from build123d import *

# Parameters (mm, degrees)
F0_W     = 38.1
F0_H     = 38.1
F1_DEPTH = 38.1
F2_W     = 38.1
F2_H     = 36.83
F3_DEPTH = 36.83
F6_DEPTH = 3.81
F7_DEPTH = 4.826


with BuildPart() as f1:
    # F0 (on Top) → F1 (new body)
    with BuildSketch(Plane.XY):
        Rectangle(F0_W, F0_H)
    extrude(amount=F1_DEPTH)

    # F2 (on face) → F3 (cut)
    with BuildSketch(Plane.XY.offset(38.1)):
        with Locations((0, -0.635)):
            Rectangle(F2_W, F2_H)
    extrude(amount=-F3_DEPTH, mode=Mode.SUBTRACT)

    # F4 (on face) → F6 (cut)
    with BuildSketch(Plane.XZ.offset(-17.78)):
        with BuildLine():
            ThreePointArc((3.96875, 19.685), (2.80633, 22.49133), (0, 23.65375))
            Line((0, 23.65375), (0, 15.71625))
            ThreePointArc((0, 15.71625), (2.80633, 16.87867), (3.96875, 19.685))
        make_face()
        with BuildLine():
            Line((0, 15.71625), (0, 23.65375))
            ThreePointArc((0, 23.65375), (-3.96875, 19.685), (0, 15.71625))
        make_face()
    extrude(amount=-F6_DEPTH, mode=Mode.SUBTRACT)

    # F5 (on face) → F7 (cut)
    with BuildSketch(Plane.XY.offset(1.27)):
        with BuildLine():
            ThreePointArc((3.96875, -0.635), (2.80633, 2.17133), (0, 3.33375))
            Line((0, 3.33375), (0, -4.60375))
            ThreePointArc((0, -4.60375), (2.80633, -3.44133), (3.96875, -0.635))
        make_face()
        with BuildLine():
            Line((0, -4.60375), (0, 3.33375))
            ThreePointArc((0, 3.33375), (-3.96875, -0.635), (0, -4.60375))
        make_face()
    extrude(amount=-F7_DEPTH, mode=Mode.SUBTRACT)


solid = f1.part
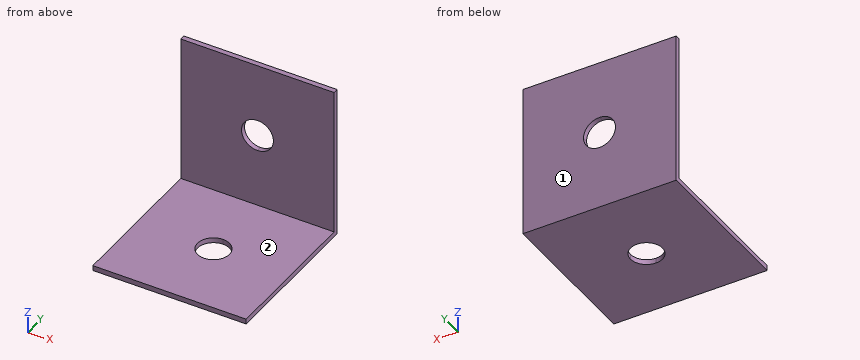
Model file for the job. Use its own axes, mm. Face numbers are marked on the shaded views. A direction names the side the tool comes from. Give positions to 0.01 mm unless a question says otherwise; leave off trailing zeros. Loops run counter-clockwise (first coordinate to the right, second up) from the corner with the lowest first, then second, coordinate; pieces in that order, holes last. Notation, with made-up numbers: (57.5, -6.5) -> (80.5, -6.5) arc R21 cw to (80.5, -2.5) -> close; hole circle Ø6 at (70, -10.75). An arc over 180 degrees is marked (long way). Use a Markdown table: item, result. Add a question column.
(1) Slice it at A-A on x = -1. List the corners of the cut face in (y, z), and give its area (3 significant figures).
(2) Drop flat-ended pins along their axis: pin 1 Ø3 at (x, y) = (12, -0.5) entering from +Z; pin 2 Ø11 at (x, z) = (-8, 23.5) entering from -Y; pin 3 Ø12 at (x, y) = (9, 15) entering from +Z. Give the stop position or say it passes through.
(3) Slice it at B-B on y = -1.5. List the corners of the cut face in (x, z), and give its area (3 significant figures).
(4) Tool access for the marked faces 1 and 2: list every direction of +Z, -Z, +X, -X, +Y, -Y with a clear straight run to the whole face (end or side of a thin tool).
(5) Wall check: line 1 along Z through (x, y) = (-8.5, -6); line 2 along Y through (x, z) = (-8.5, 24.5). Give the ranges that are in metal, low to high.
(6) Slice it at C-C on z = 17. List the corners of the cut face in (x, y).
(7) Slice it at D-D on x = 5. List the corners of the cut face in (y, z).
Filled sheet:
| question | item | result |
|---|---|---|
| 1 | outline | (-19.05, 0) -> (-4.48, 0) -> (-4.48, 1.27) -> (-19.05, 1.27) -> close; (3.21, 0) -> (19.05, 0) -> (19.05, 15.84) -> (17.78, 15.84) -> (17.78, 1.27) -> (3.21, 1.27) -> close; (17.78, 23.53) -> (19.05, 23.53) -> (19.05, 38.1) -> (17.78, 38.1) -> close |
| 1 | area | 75.7 mm2 |
| 2 | pin 1 | z = 1.27 |
| 2 | pin 2 | y = 17.78 |
| 2 | pin 3 | z = 38.1 |
| 3 | outline | (-19.05, 0) -> (-3.87, 0) -> (-3.87, 1.27) -> (-19.05, 1.27) -> close; (3.87, 0) -> (19.05, 0) -> (19.05, 1.27) -> (3.87, 1.27) -> close |
| 3 | area | 38.5 mm2 |
| 4 | face 1 | +Z, -Z, +X, -X, +Y |
| 4 | face 2 | +Z, +X, -X, -Y |
| 5 | line 1 | 0 to 1.27 |
| 5 | line 2 | 17.78 to 19.05 |
| 6 | outline | (-19.05, 17.78) -> (-2.92, 17.78) -> (-2.92, 19.05) -> (-19.05, 19.05) -> close; (2.92, 17.78) -> (19.05, 17.78) -> (19.05, 19.05) -> (2.92, 19.05) -> close |
| 7 | outline | (-19.05, 0) -> (19.05, 0) -> (19.05, 38.1) -> (17.78, 38.1) -> (17.78, 1.27) -> (-19.05, 1.27) -> close |
